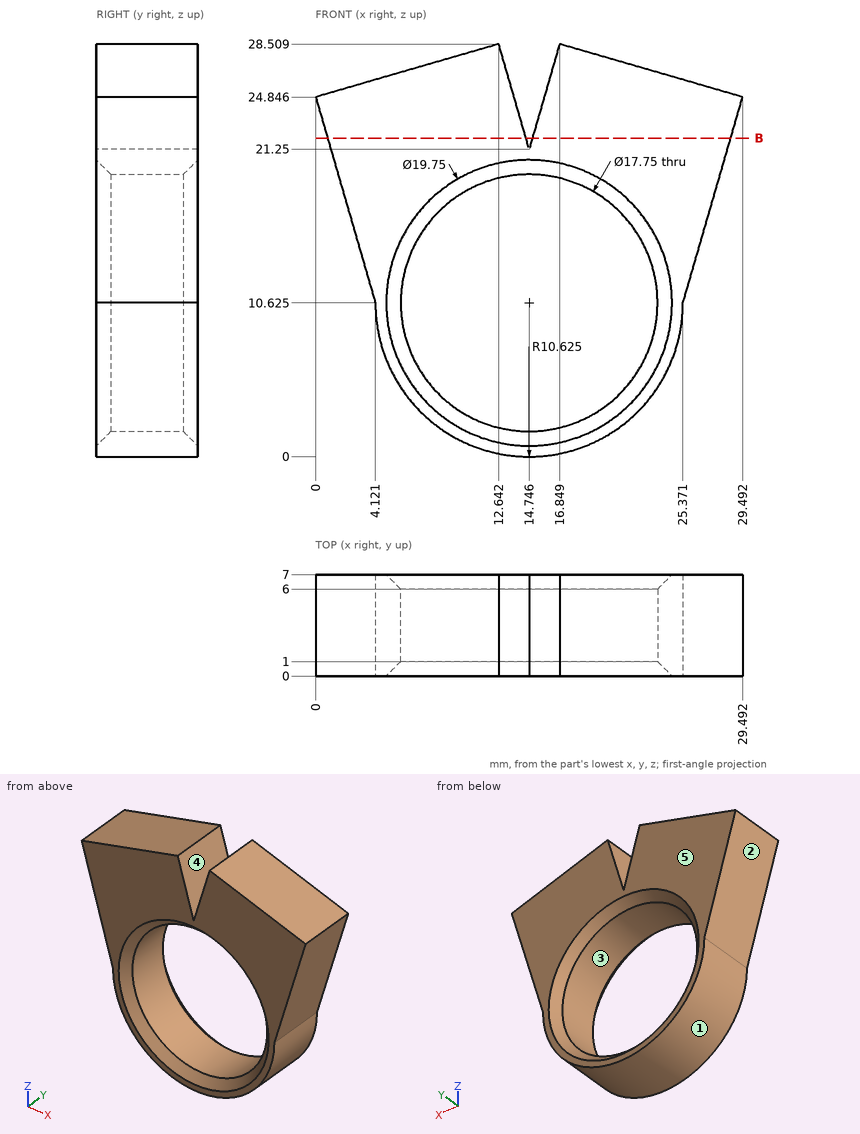
Drawing for the job (mm, zero at the part's lowest x, y, z). A direction names the side the tool comes from. Give positions to 0.01 mm unless a question says otherwise; leave off trailing zeros. Loops run counter-clockwise (first coordinate to the right, second up) from the corner with the lowest first, then second, coordinate; pieces in that order, holes last. Notation, with made-up numbers: M 58,29.5 L 90,29.5 A11 cw 90,35.5 Z; hole C 87,68 d1. An arc over 180 degrees is marked long. Use one line per item in the form item = value.
Item 1: Flat gauge pin, fed straight in: pin 1 (4 mm diameter, centred on y = 4, z = 3, fed in from +X). Where does the tip first touch, or does it go through?
Determined:
pin_1 = 23.76
Item 2: Which spindle directions (+Z, -Z, +X, -X, +Y, -Y) get a long thin tool onto all of the face, cutting with end or side? Do the marked faces 4 and 5. Say none if no direction does.
Determined:
face_4 = +Z, +Y, -Y
face_5 = +Z, -Z, +X, -X, +Y
Item 3: Slice it at B-B (z = 22). List the corners of the cut face in (x, y) (1 decimal).
Determined:
outline = M 0.8,0 L 14.5,0 L 14.5,7 L 0.8,7 Z; M 15,0 L 28.7,0 L 28.7,7 L 15,7 Z
Item 4: Two-plate mould, pull along X, no slides. Class the marked faces 1, 2 and 3: pulls with the +X half, pulls with the -X half, needs draft (parallel to the pull), parting line crosses it, or undercut.
Determined:
face_1 = parting line crosses it
face_2 = pulls with the -X half
face_3 = undercut
Item 5: Drill centre lines: probe 1 along X at (y, z) = (2.5, 7) (1 decimal); probe 2 along Z at (x, y) = (10, 3.75) (1 decimal); probe 3 along Z at (x, y) = (8.5, 3.5). Where is each one in solid material? Low to high. Write a range as from..to.
Determined:
probe_1 = 4.8..6.6, 22.8..24.7
probe_2 = 1.1..3.1, 18.1..27.7
probe_3 = 2.03..4.32, 16.93..27.31
